Check sheet for the modelled part. Datum: model origin and axes. Units: mm. Give positions to 0.01 mm unless a question says otherwise; leave off trailing zeros. Order: outer loops, then holes, each group sorted by start corner. A loop starts at its lowest first (then second) coordinate and runs counter-clockwise, first axis right, second up.
```python
from build123d import *

# Parameters (mm, degrees)
SKETCH1_W           = 12.7
SKETCH1_H           = 12.7
SKETCH1_R           = 1.905
BOSS_EXTRUDE1_DEPTH = 88.9
SKETCH3_W           = 12.7
SKETCH3_H           = 17.145
SKETCH3_R           = 2.286
BOSS_EXTRUDE2_DEPTH = 28.575
SKETCH4_W           = 12.7
SKETCH4_H           = 17.145
CUT_EXTRUDE1_DEPTH  = 13.97
FILLET1_R           = 2.54


with BuildPart() as part:
    # Sketch1 → Boss-Extrude1 (new, symmetric)
    # profile 1 of 2: a face of its own
    with BuildSketch(Plane.XY):
        with Locations((-6.35, -6.35)):
            Rectangle(SKETCH1_W, SKETCH1_H)
        with Locations((-6.35, -6.35)):
            Circle(SKETCH1_R, mode=Mode.SUBTRACT)
    # profile 2 of 2: a face of its own
    with BuildSketch(Plane.XY):
        with Locations((-6.35, 6.35)):
            Rectangle(SKETCH1_W, SKETCH1_H)
        with Locations((-6.35, 6.35)):
            Circle(SKETCH1_R, mode=Mode.SUBTRACT)
    extrude(amount=BOSS_EXTRUDE1_DEPTH, both=True)

    # Sketch3 → Boss-Extrude2 (add, symmetric)
    with BuildSketch(Plane.XY):
        with Locations((-6.35, 21.2725)):
            Rectangle(SKETCH3_W, SKETCH3_H)
        with Locations((-6.35, 23.495)):
            Circle(SKETCH3_R, mode=Mode.SUBTRACT)
    extrude(amount=BOSS_EXTRUDE2_DEPTH, both=True)

    # Sketch4 → Cut-Extrude1 (cut, symmetric)
    with BuildSketch(Plane.XY):
        with Locations((-6.35, 21.2725)):
            Rectangle(SKETCH4_W, SKETCH4_H)
    extrude(amount=CUT_EXTRUDE1_DEPTH, both=True, mode=Mode.SUBTRACT)

    # Fillet1
    fillet1_edges = [part.edges().sort_by_distance(p)[0] for p in [
        (0, -12.7, 0),
        (-12.7, -12.7, 0),
        (-12.7, 12.7, -58.7375),
        (0, 12.7, -58.7375),
        (0, 12.7, 58.7375),
        (-12.7, 12.7, 58.7375),
        (0, 29.845, 21.2725),
        (-12.7, 29.845, 21.2725),
        (-12.7, 29.845, -21.2725),
        (0, 29.845, -21.2725),
        (-12.7, 12.7, 0),
        (0, 12.7, 0),
    ]]
    fillet(fillet1_edges, radius=FILLET1_R)


solid = part.part
```
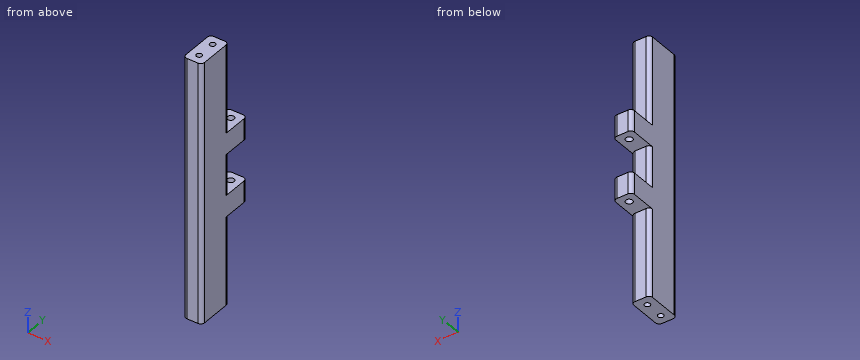
(1) Gauge pin test, flat ends, axial feed: pin 1 Ø4 at (x, y) = (-8, 19.5) entering from +Z (3 decimals); pin 2 Ø1.5 at (x, z) = (-4.5, 0) entering from +Y; pin 3 Ø4 at (x, y) = (-7, 17) entering from -Z (3 decimals). Record the tip position at first contact, or that the pin passes through.
Response values:
pin 1: stops at z = 28.575
pin 2: stops at y = 12.7
pin 3: stops at z = -28.575
(2) Material ranges on L1, parallel to Y at x = -6.35, z = -22.5 (3 decimals); L2, parallel to Y at x = -6, z = 1.5; L3, parallel to Y at x = -6.35, z = 2 (3 decimals), recorded low to high.
Response values:
L1: y = -12.7 to -8.255, -4.445 to 4.445, 8.255 to 21.209, 25.781 to 29.845
L2: y = -12.7 to -8.22, -4.48 to 4.48, 8.22 to 12.7
L3: y = -12.7 to -8.255, -4.445 to 4.445, 8.255 to 12.7
(3) Cross-section at A-A on y = -6.35. Enter the section's corners in (x, z) (3 decimals), then the cut area to 3 significant figures.
Response values:
outline: (-12.7, -88.9) - (-8.255, -88.9) - (-8.255, 88.9) - (-12.7, 88.9) - close; (-4.445, -88.9) - (0, -88.9) - (0, 88.9) - (-4.445, 88.9) - close
area: 1,580 mm2
(4) Cross-section at C-C on z = 6.5. Enter the section's corners in (x, y) (3 decimals), then the cut area to 3 significant figures.
Response values:
outline: (-12.7, -10.16) arc R2.54 ccw to (-10.16, -12.7) - (-2.54, -12.7) arc R2.54 ccw to (0, -10.16) - (0, 10.16) arc R2.54 ccw to (-2.54, 12.7) - (-10.16, 12.7) arc R2.54 ccw to (-12.7, 10.16) - close; hole circle Ø3.81 at (-6.35, -6.35); hole circle Ø3.81 at (-6.35, 6.35)
area: 294 mm2
(5) Cross-section at B-B on x = -6.35. Enter the section's corners in (y, z) (3 decimals).
Response values:
outline: (-12.7, -88.9) - (-8.255, -88.9) - (-8.255, 88.9) - (-12.7, 88.9) - close; (-4.445, -88.9) - (4.445, -88.9) - (4.445, 88.9) - (-4.445, 88.9) - close; (8.255, -88.9) - (12.7, -88.9) - (12.7, -28.575) - (21.209, -28.575) - (21.209, -13.97) - (12.7, -13.97) - (12.7, 13.97) - (21.209, 13.97) - (21.209, 28.575) - (12.7, 28.575) - (12.7, 88.9) - (8.255, 88.9) - close; (25.781, -28.575) - (29.845, -28.575) - (29.845, -13.97) - (25.781, -13.97) - close; (25.781, 13.97) - (29.845, 13.97) - (29.845, 28.575) - (25.781, 28.575) - close
